from build123d import *

# Parameters (mm, degrees)
SKETCH1_W           = 120
SKETCH1_H           = 160
BOSS_EXTRUDE1_DEPTH = 3
SKETCH2_R           = 1.5
CUT_EXTRUDE12_DEPTH = 3
SKETCH3_R           = 1.5
CUT_EXTRUDE13_DEPTH = 10


with BuildPart() as part:
    # Sketch1 → Boss-Extrude1 (new body)
    with BuildSketch(Plane(origin=(0, 0, 0), x_dir=(1, 0, 0), z_dir=(0, 1, 0))):
        with Locations((-60, 80)):
            Rectangle(SKETCH1_W, SKETCH1_H)
    extrude(amount=BOSS_EXTRUDE1_DEPTH)

    # Sketch2 → Cut-Extrude12 (cut)
    with BuildSketch(Plane(origin=(0, 3, 0), x_dir=(1, 0, 0), z_dir=(0, 1, 0))):
        with Locations(Location((-25, 112.75, 0), (0, 0, 270))):
            Circle(SKETCH2_R)
        with Locations(Location((-3.5, 105.75, 0), (0, 0, 270))):
            Circle(SKETCH2_R)
        with Locations(Location((-34, 136.75, 0), (0, 0, 270))):
            Circle(SKETCH2_R)
        with Locations(Location((-25, 136.75, 0), (0, 0, 270))):
            Circle(SKETCH2_R)
        with Locations(Location((-34, 112.75, 0), (0, 0, 270))):
            Circle(SKETCH2_R)
        with Locations(Location((-3.5, 142.75, 0), (0, 0, 270))):
            Circle(SKETCH2_R)
        with Locations(Location((-12, 148, 0), (0, 0, 270))):
            Circle(SKETCH2_R)
        with Locations(Location((-12, 153, 0), (0, 0, 270))):
            Circle(SKETCH2_R)
        with Locations(Location((-108, 153, 0), (0, 0, 90))):
            Circle(SKETCH2_R)
        with Locations(Location((-108, 148, 0), (0, 0, 90))):
            Circle(SKETCH2_R)
        with Locations(Location((-116.5, 142.75, 0), (0, 0, 90))):
            Circle(SKETCH2_R)
        with Locations(Location((-95, 136.75, 0), (0, 0, 90))):
            Circle(SKETCH2_R)
        with Locations(Location((-86, 136.75, 0), (0, 0, 90))):
            Circle(SKETCH2_R)
        with Locations(Location((-86, 112.75, 0), (0, 0, 90))):
            Circle(SKETCH2_R)
        with Locations(Location((-95, 112.75, 0), (0, 0, 90))):
            Circle(SKETCH2_R)
        with Locations(Location((-116.5, 105.75, 0), (0, 0, 90))):
            Circle(SKETCH2_R)
        with Locations(Location((-3.5, 47.75, 0), (0, 0, 270))):
            Circle(SKETCH2_R)
        with Locations(Location((-3.5, 10.75, 0), (0, 0, 270))):
            Circle(SKETCH2_R)
        with Locations(Location((-116.5, 47.75, 0), (0, 0, 90))):
            Circle(SKETCH2_R)
        with Locations(Location((-116.5, 10.75, 0), (0, 0, 90))):
            Circle(SKETCH2_R)
    extrude(amount=-CUT_EXTRUDE12_DEPTH, mode=Mode.SUBTRACT)

    # Sketch3 → Cut-Extrude13 (cut)
    with BuildSketch(Plane(origin=(0, 3, 0), x_dir=(1, 0, 0), z_dir=(0, 1, 0))):
        with Locations(Location((-117, 157, 0), (0, 0, 270))):
            Circle(SKETCH3_R)
        with Locations(Location((-3, 157, 0), (0, 0, 270))):
            Circle(SKETCH3_R)
        with Locations(Location((-117, 3, 0), (0, 0, 270))):
            Circle(SKETCH3_R)
        with Locations(Location((-3, 3, 0), (0, 0, 270))):
            Circle(SKETCH3_R)
    extrude(amount=-CUT_EXTRUDE13_DEPTH, mode=Mode.SUBTRACT)


solid = part.part
For this review, take the finished solid that the model builds, in its own axes (mm). Round coordinates to 2 decimals unless told otherwise and drop trailing zeros. Write item = value, one per line. Start each with the question number.
1) Insertion check: pin 1 (2.5 mm diameter, centred on x = -34, z = -136.75, fed in from -Y). The pin has a flat end and moves straight along its axis. Give the tip position at first contact, or say it passes through.
2) The part is to be moulded in two halves that separate along Y. For faces 1 (the face through (-61, 0, -81)), 2 (the face through (-61, 3, -81)), say which applies: +Y half, -Y half, draft (parallel to the pull), parting line (faces both ways), or undercut.
3) To check wall thickness, follow line 1 (Z direction, x = -108, y = 1.35); line 2 (X direction, y = 1.65, z = -153); line 3 (X direction, y = 2.75, z = -106). State the ranges of each line that lie inside material, in increasing order. Write a range as from..to.
Verdict:
q1.pin_1 = through
q2.face_1 = -Y half
q2.face_2 = +Y half
q3.line_1 = -160..-154.5, -151.5..-149.5, -146.5..0
q3.line_2 = -120..-109.5, -106.5..-13.5, -10.5..0
q3.line_3 = -120..-117.98, -115.02..-4.98, -2.02..0
